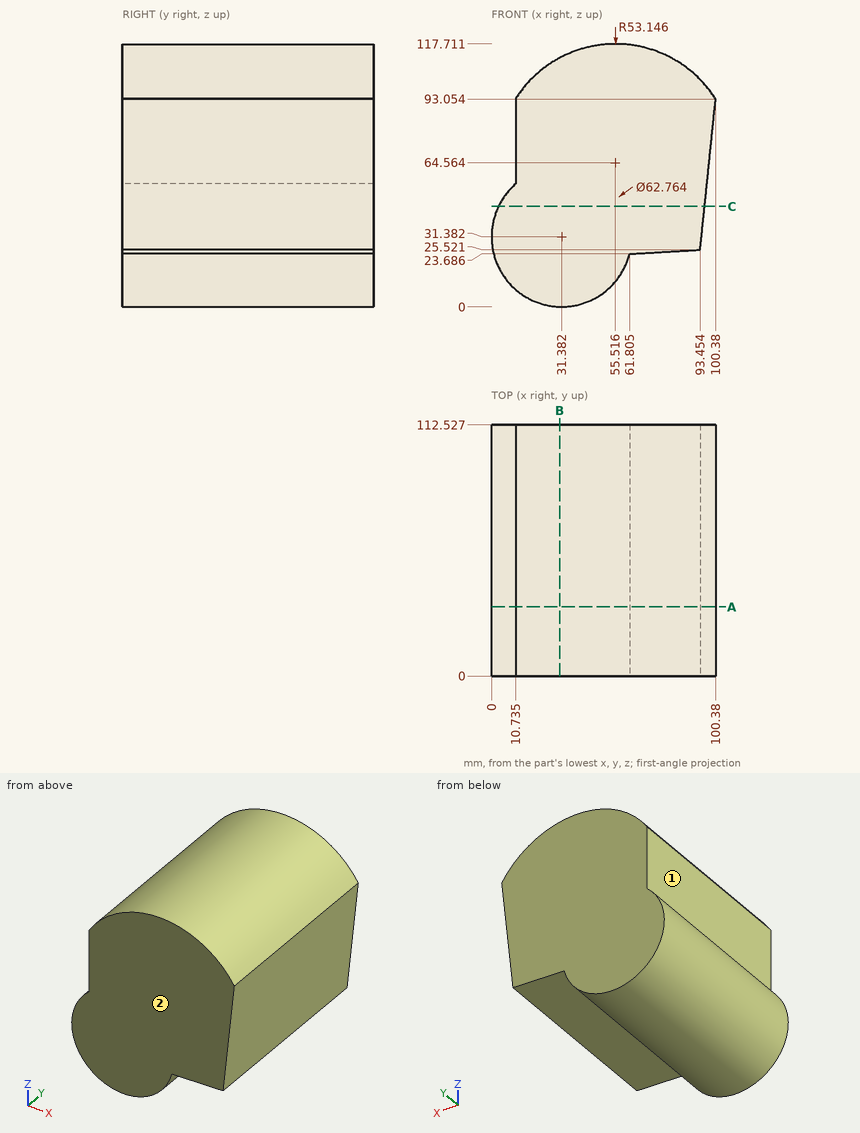
Check sheet for the drawn part. Datum: minimum x, y, z corner. Units: mm. A direction names the side the tool comes from. Give positions to 0.01 mm unless a question says otherwise; leave off trailing zeros. Order: outer loops, then holes, each group sorted by start corner. A loop starts at its lowest first (then second) coordinate and runs counter-clockwise, first axis right, second up. Notation, with made-up numbers: (75, 47.25) - (85, 47.25) arc R14 ccw to (85, 65.25) - close; hole circle Ø8 at (25.5, -1.75). An arc over 180 degrees is marked (long way). Answer in a Markdown table with one row per item. Add a question column.
Q1. Material ranges on probe 1 along X at (y, z) = (6.5, 105.5); probe 2 along Z at (x, y) = (90, 42) (1 decimal); probe 3 along X at (y, z) = (17, 41), recorded low to high. Write a range as from..to.
Q2. Cross-section at C-C, the plane z = 45. Enter the section's corners in (x, y).
Q3. Tool access check on the marked faces 1 and 2. Record the directions out of +Z, -Z, +X, -X, +Y, -Y that give a thin tool (end or side, any length) a straight path to the whole face; none if there is none.
Q4. Cross-section at B-B, the plane x = 30.5. Enter the section's corners in (y, z) (1 decimal), then the cut area to 3 significant figures.
Q5. Gauge pin test, flat ends, axial feed: pin 1 (6 mm diameter, centred on x = 83.5, y = 80, fed in from -Z); pin 2 (2 mm diameter, centred on y = 95.5, z = 24.5, fed in from -X); pin 3 (3 mm diameter, centred on x = 60, y = 29, fed in from +Z). Record the tip position at first contact, or that the pin passes through.
Q6. Cross-section at A-A, the plane y = 31. Enter the section's corners in (x, z) (1 decimal).
Check values:
| question | item | result |
|---|---|---|
| 1 | probe 1 | x = 21.62..89.41 |
| 1 | probe 2 | z = 25.3..105 |
| 1 | probe 3 | x = 1.51..95.04 |
| 2 | outline | (3.11, 0) - (95.45, 0) - (95.45, 112.53) - (3.11, 112.53) - close |
| 3 | face 1 | +Z, -X, +Y, -Y |
| 3 | face 2 | +Z, -Z, +X, -X, -Y |
| 4 | outline | (0, 0) - (112.5, 0) - (112.5, 111.5) - (0, 111.5) - close |
| 4 | area | 12,500 mm^2 |
| 5 | pin 1 | stops at z = 24.77 |
| 5 | pin 2 | stops at x = 0.56 |
| 5 | pin 3 | stops at z = 117.63 |
| 6 | outline | (10.7, 55) arc R31.4 ccw (long way) to (61.8, 23.7) - (93.5, 25.5) - (100.4, 93.1) arc R53.1 ccw to (10.7, 93.2) - close |
